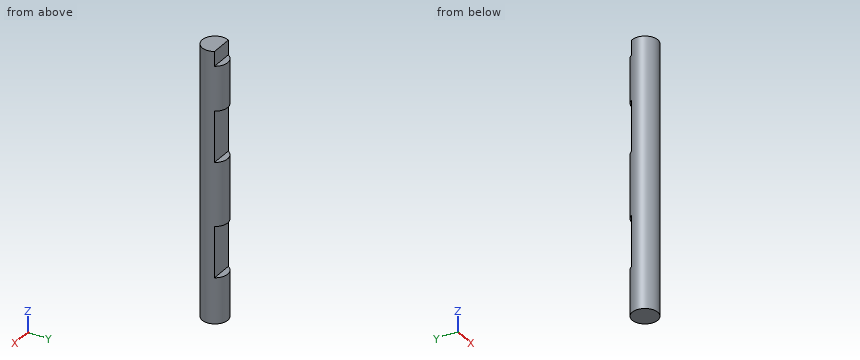
Autodesk Inventor part; units mm, degrees
ref_plane "YZ Plane" through (0, 0, 0) normal (1, 0, 0) x (0, 1, 0)
ref_plane "XZ Plane" through (0, 0, 0) normal (0, 1, 0) x (-1, 0, 0)
ref_plane "XY Plane" through (0, 0, 0) normal (0, 0, 1) x (1, 0, 0)
sketch "スケッチ1" plane through (0, 0, 0) normal (0, 0, 1) x (1, 0, 0)
  circle A0 centre (0, 0) radius 2
  dimension "d0" = 4
extrude "押し出し1" add sketch "スケッチ1" along normal blind 42.5
sketch "スケッチ2" plane through (0, 0, 42.5) normal (0, 0, 1) x (1, 0, 0)
  circle A0 centre (0, 0) radius 2
  line L0 (-1.7321, 1) -> (1.7321, 1)
  dimension "d3" = 1
extrude "押し出し2" cut sketch "スケッチ2" against normal blind 2.3 contours L0 A0 picked at (0.4849, 1.1242)
sketch "スケッチ3" plane through (0, 0, 42.5) normal (0, 0, 1) x (1, 0, 0)
  point P0 (0, 0)
sketch "スケッチ4" plane through (0, 0, 0) normal (0, 0, -1) x (-1, 0, 0)
  arc A0 (1.7321, 1) -> (-1.7321, 1) centre (0, 0) ccw
  circle A1 centre (0, 0) radius 2
sketch "スケッチ5" plane through (-1.7321, 1, 42.5) normal (0, 1, 0) x (1, 0, 0)
  point P0 (1.7321, 42.5)
sketch "スケッチ6" plane through (-1.7321, 1, 42.5) normal (0, 1, 0) x (1, 0, 0)
  line L0 (-15.0722, 17.3) -> (4.9278, 17.3)
  line L1 (4.9278, 17.3) -> (4.9278, 9.3)
  line L2 (4.9278, 9.3) -> (-15.0722, 9.3)
  line L3 (-15.0722, 9.3) -> (-15.0722, 17.3)
  line L4 (3.4641, 2.3) -> (0, 2.3)
  line L5 (-8.306, 35.3) -> (11.694, 35.3)
  line L6 (11.694, 35.3) -> (11.694, 27.3)
  line L7 (11.694, 27.3) -> (-8.306, 27.3)
  line L8 (-8.306, 27.3) -> (-8.306, 35.3)
  point P0 (1.7321, 42.5)
  dimension "d8" = 8
  dimension "d9" = 20
  dimension "d10" = 15
  dimension "d12" = 20
  dimension "d13" = 25
  dimension "d16" = 8
extrude "押し出し3" cut sketch "スケッチ6" along normal blind 10
properties part number "3SR03_振子軸"
Geometry check sheet. Reference: the model listing, model coordinates, mm. Round coordinates to 2 decimals unless told otherwise and drop trailing zeros. Order: outer loops, then holes, each group sorted by start corner. A loop starts at its lowest first (then second) coordinate and runs counter-clockwise, first axis right, second up. Notation, with made-up numbers: M -36.5,8.25 L -19.5,8.25 A32 ccw -19.5,42.25 Z; hole C 77,62.5 d7. An arc over 180 degrees is marked long. Answer in a Markdown table with one row per item.
(1) Go/stop test with flat-tipped pins: P1, Ø0.5, axis at x = 0.5, y = 1.5, coming from the +Z side; P2, Ø1, axis at y = 1.5, z = 21.5, coming from the +X side; P3, Ø0.7, axis at x = 1, z = 41, coming from the +Y side. Record where each tip stops, or that it passes through.
Responses:
| item | result |
|---|---|
| P1 | stops at z = 40.2 |
| P2 | stops at x = 1.73 |
| P3 | stops at y = 1 |
(2) Scan lines: probe 1 along Z at (x, y) = (-0.9, 1.75); probe 2 along Y at (x, z) = (-1.45, 6); probe 3 along Y at (x, z) = (1.2, 3.5). Record each from-to range of solid material in increasing order. Write a range as from..to.
Responses:
| item | result |
|---|---|
| probe 1 | z = 0..7.2, 15.2..25.2, 33.2..40.2 |
| probe 2 | y = -1.38..1.38 |
| probe 3 | y = -1.6..1.6 |
(3) Sectioned sample at A-A, the plane x = 0. Record the cut outline in (y, z), and give its area (3 significant figures).
Responses:
| item | result |
|---|---|
| outline | M -2,0 L 2,0 L 2,7.2 L 1,7.2 L 1,15.2 L 2,15.2 L 2,25.2 L 1,25.2 L 1,33.2 L 2,33.2 L 2,40.2 L 1,40.2 L 1,42.5 L -2,42.5 Z |
| area | 152 mm² |
(4) Sectioned sample at B-B, the plane z = 11.5. Record the cut outline in (x, y).
Responses:
| item | result |
|---|---|
| outline | M -1.73,1 A2 ccw long 1.73,1 Z |
(5) Sectioned sample at C-C, the plane y = -1.45. Record the cut outline in (x, z).
Responses:
| item | result |
|---|---|
| outline | M -1.38,0 L 1.38,0 L 1.38,42.5 L -1.38,42.5 Z |
(6) Sectioned sample at D-D, the plane z = 3.5. Record the cut outline in (x, y), and give its area (3 significant figures).
Responses:
| item | result |
|---|---|
| outline | C 0,0 d4 |
| area | 12.6 mm² |
